For this review, take the finished solid that the model builds, in its own axes (mm). A direction names the side the tool comes from. Give positions to 0.01 mm unless a question says otherwise; leave off trailing zeros. Loops run counter-clockwise (first coordinate to the right, second up) from the corner with the lowest first, then second, coordinate; pieces in that order, holes last. Notation, with made-up numbers: (49, -3.75) - (79, -3.75) arc R8 cw to (79, 4.25) - close; hole circle Ø8 at (78.25, 43). An arc over 180 degrees is marked (long way). Answer as CSV lines item,"result".
from build123d import *

# Parameters (mm, degrees)
EXTRUDE_1_DEPTH = 40


with BuildPart() as part:
    # 草图1 → 凸台-拉伸1 (new body)
    with BuildSketch(Plane(origin=(0, 0, 0), x_dir=(1, 0, 0), z_dir=(0, 1, 0))):
        with BuildLine():
            Line((0, -8), (0, -75))
            Line((0, -75), (6, -75))
            Line((6, -75), (6, -14))
            ThreePointArc((6, -14), (8.343145751, -8.343145751), (14, -6))
            Line((14, -6), (92, -6))
            Line((92, -6), (92, 0))
            Line((92, 0), (8, 0))
            ThreePointArc((8, 0), (2.343145751, -2.343145751), (0, -8))
        make_face()
    extrude(amount=EXTRUDE_1_DEPTH)


solid = part.part
1) Insertion check: P1, Ø1.5, axis at x = 33, y = 19.5, coming from the -Z side; P2, Ø20, axis at y = 14, z = 39, coming from the +X side; P3, Ø12, axis at x = 36.5, y = 20.5, coming from the +Z side. Each pin has a flat end and moves straight along its axis. Give the tip position at first contact, or say it passes through.
From the geometry:
P1,"stops at z = 0"
P2,"stops at x = 6"
P3,"stops at z = 6"
2) Consider section C-C on z = 66. Write out the cut boundary in (x, y).
From the geometry:
outline,"(0, 0) - (6, 0) - (6, 40) - (0, 40) - close"
3) Consider section B-B on x = 48. Write out the cut boundary in (y, z), and give its area (3 significant figures).
From the geometry:
outline,"(0, 0) - (40, 0) - (40, 6) - (0, 6) - close"
area,"240 mm^2"
4) Consider section A-A on y = 12. Write out the cut boundary in (x, z).
From the geometry:
outline,"(0, 8) arc R8 ccw to (8, 0) - (92, 0) - (92, 6) - (14, 6) arc R8 cw to (6, 14) - (6, 75) - (0, 75) - close"
5) Wall thickness on line 1 (Z direction, x = 53.5, y = 18.5); line 2 (X direction, y = 14.5, z = 9) (3 decimals): over which ranges is each line inside the solid? List them lowest first. Write a range as from..to.
From the geometry:
line 1,"z = 0..6"
line 2,"x = 0..7.755"
6) Machinability: for faces 1 (the flat face through (51, 20, 0)), 2 (the flat face through (52, 20, 6)), which of the approach directions +Z, -Z, +X, -X, +Y, -Y give a long, thin tool a straight path to every point of the face, cutting with its end or side? Answer none if there is none.
From the geometry:
face 1,"-Z, +X, -X, +Y, -Y"
face 2,"+Z, +X, +Y, -Y"
